Read the model definition and answer for the solid it produces. Units are mm, in the model's axes. Face numbers are marked on the shaded views. A direction names the side the tool comes from. Give positions to 0.01 mm unless a question says otherwise; leave off trailing zeros. Order: outer loops, then holes, each group sorted by start corner. A loop starts at its lowest first (then second) coordinate and runs counter-clockwise, first axis right, second up. Notation, with made-up numbers: (26.5, 63) -> (45.5, 63) arc R21 ccw to (45.5, 88) -> close; hole circle Ø2 at (15.5, 8.25). An arc over 180 degrees is marked (long way). Answer as CSV lines item,"result". Start each with the question number.
1) The mould has two halves that part along X. Classify the marked faces 4, 5, 6 and 7: +X half, -X half, draft (parallel to the pull), parting line (faces both ways), or undercut.
2) Find section A-A (y = 31.5). Determine the outline of the cut face in (x, z).
3) Flat-ended cylindrical pins translate along their axes: pin 1 Ø6 at (x, y) = (-9.5, 11) entering from +Z; pin 2 Ø12 at (x, y) = (-13, 20) entering from -Z; pin 3 Ø6 at (y, z) = (41, 6.5) entering from +X. Find the tip coordinate at first contact, or state that the pin passes through.
4) For the marked faces 1, 2 and 3, determine the directions among +Z, -Z, +X, -X, +Y, -Y from which every point of the face is accessible in a straight line to the end or side of a thin tool.
5) Straight lines are drawn through the part: L1, parallel to X at y = 10.5, z = -1; L2, parallel to Y at x = -4, z = 14.5. For each, find the intervals that lie inside material, in ascending order. Write a range as from..to.
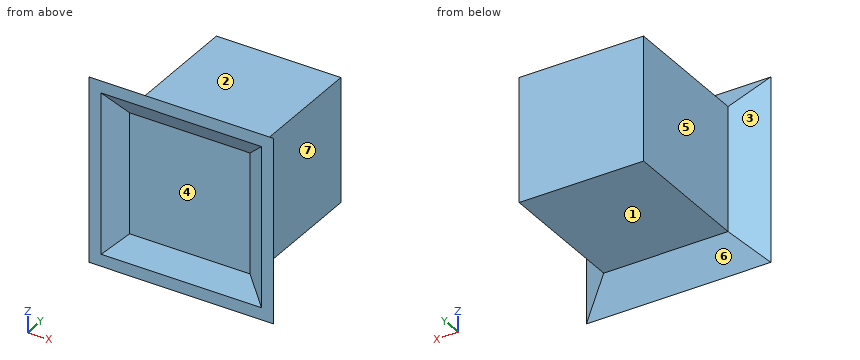
```python
from build123d import *

# Parameters (mm, degrees)
SHELL4_T            = 2
SKETCH8_W           = 37.21110255
SKETCH8_H           = 37.21110255
BOSS_EXTRUDE1_DEPTH = 40


with BuildPart() as part:
    # Sketch1 → Loft1 section 0
    with BuildSketch(Plane(origin=(0, 0, 0), x_dir=(1, 0, 0), z_dir=(0, 1, 0))):
        with BuildLine():
            Line((-24, 24), (24, 24))
            Line((24, 24), (24, -24))
            Line((24, -24), (-24, -24))
            Line((-24, -24), (-24, 24))
        make_face()
    # Sketch2 → Loft1 section 1
    with BuildSketch(Plane(origin=(0, 4, 0), x_dir=(1, 0, 0), z_dir=(0, 1, 0))):
        with BuildLine():
            Line((-18, 18), (18, 18))
            Line((18, 18), (18, -18))
            Line((18, -18), (-18, -18))
            Line((-18, -18), (-18, 18))
        make_face()
    loft()

    # Shell4
    shell4_openings = [part.faces().sort_by_distance(p)[0] for p in [
        (0, 0, 0),
    ]]
    offset(amount=SHELL4_T, openings=shell4_openings, kind=Kind.INTERSECTION)

    # Sketch8 → Boss-Extrude1 (add)
    with BuildSketch(Plane(origin=(0, 6, 0), x_dir=(1, 0, 0), z_dir=(0, 1, 0))):
        Rectangle(SKETCH8_W, SKETCH8_H)
    extrude(amount=BOSS_EXTRUDE1_DEPTH)


solid = part.part
```
Findings below:
1,face 4,"undercut"
1,face 5,"-X half"
1,face 6,"draft"
1,face 7,"+X half"
2,outline,"(-18.61, -18.61) -> (18.61, -18.61) -> (18.61, 18.61) -> (-18.61, 18.61) -> close"
3,pin 1,"z = 18.61"
3,pin 2,"z = -18.61"
3,pin 3,"x = 18.61"
4,face 1,"-Z, +X, -X, +Y"
4,face 2,"+Z, +X, -X, +Y"
4,face 3,"+Z, -Z, -X, +Y"
5,L1,"-18.61..18.61"
5,L2,"4..46"
